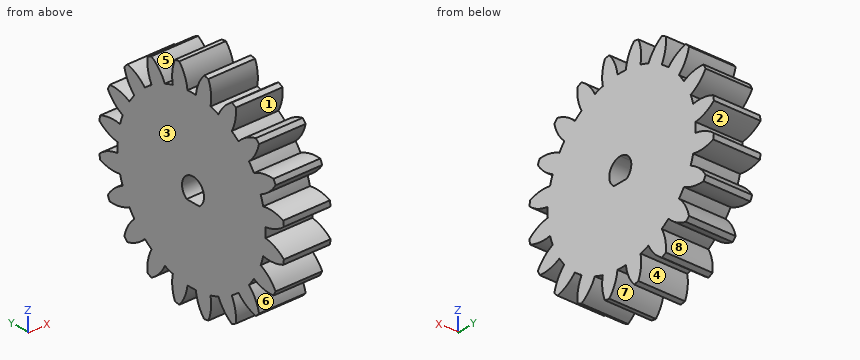
```python
from build123d import *

# Parameters (mm, degrees)
BASPROSKE_W           = 12
BASPROSKE_H           = 27.5
TOOTHCUT_DEPTH        = 41.70012285
TEETHCUTS_COUNT       = 20
TEETHCUTS_ANGLE       = 342
BORSKE_R              = 0.4
BORE_DEPTH            = 50.0000508
KES_EKSTR_ZYON1_DEPTH = 100


with BuildPart() as part:
    # BasProSke → Base-Revolve (revolve)
    with BuildSketch(Plane(origin=(0, 0, 0), x_dir=(1, 0, 0), z_dir=(0, 1, 0)), mode=Mode.PRIVATE) as base_revolve_sk:
        with Locations((6, 13.75)):
            Rectangle(BASPROSKE_W, BASPROSKE_H)
    revolve(base_revolve_sk.sketch.rotate(Axis((-10, 0, 0), (1, 0, 0)), 180), axis=Axis((-10, 0, 0), (1, 0, 0)))

    # TooCutSke → ToothCut (cut, through all)
    with BuildSketch(Plane(origin=(0, 0, 0), x_dir=(0, 0, -1), z_dir=(1, 0, 0))):
        with BuildLine():
            ThreePointArc((1.237725267, 21.838954008), (0, 21.874), (-1.237725267, 21.838954008))
            ThreePointArc((-1.237725267, 21.838954008), (-2.037783758, 24.744650423), (-3.667234079, 27.280011719))
            ThreePointArc((-3.667234079, 27.280011719), (0, 27.5254), (3.667234079, 27.280011719))
            ThreePointArc((3.667234079, 27.280011719), (2.037783758, 24.744650423), (1.237725267, 21.838954008))
        make_face()
    toothcut = extrude(amount=TOOTHCUT_DEPTH, mode=Mode.SUBTRACT)

    # TeethCuts: ToothCut ×20 about axis
    teethcuts_axis = Axis((-10, 0, 0), (1, 0, 0))
    for i in range(1, TEETHCUTS_COUNT):
        add(toothcut.rotate(teethcuts_axis, i * TEETHCUTS_ANGLE / (TEETHCUTS_COUNT - 1)), mode=Mode.SUBTRACT)

    # BorSke → Bore (cut, symmetric)
    with BuildSketch(Plane(origin=(0, 0, 0), x_dir=(0, 0, -1), z_dir=(1, 0, 0))):
        with Locations(Location((0, 0, 0), (0, 0, 180))):
            Circle(BORSKE_R)
    extrude(amount=BORE_DEPTH, both=True, mode=Mode.SUBTRACT)

    # Çizim1 → Kes-Ekstrüzyon1 (cut)
    with BuildSketch(Plane.ZY):
        with BuildLine():
            ThreePointArc((3.25, -0.4), (0.99239773, 2.694777334), (-2.643936459, 1.49))
            Line((-2.643936459, 1.49), (-2.643936459, -2.29))
            ThreePointArc((-2.643936459, -2.29), (0.99239773, -3.494777334), (3.25, -0.4))
        make_face()
    extrude(amount=-KES_EKSTR_ZYON1_DEPTH, mode=Mode.SUBTRACT)


solid = part.part
```
Can you work these out from the model? Positions are in its coordinate system, mm. Face numbers are marked on the shaded views. A direction names the side the tool comes from. Round coordinates to 2 decimals unless told otherwise and drop trailing zeros. Loops run counter-clockwise (first coordinate to the right, second up) from the corner with the lowest first, then second, coordinate; pieces in that order, holes last.
Item 1: Which directions (+Z, -Z, +X, -X, +Y, -Y) give clear straight access to the entire face, cutting with the end or side of a thin tool? Please do the marked faces 5, 6, 7 and 8.
Item 2: Suppose I cut it at B-B, the plane y = 15. Write out the boundary of the cut face in (x, z), then the cut area to 3 significant figures.
Item 3: Please list where these lines run through material, in increasing order: L1, parallel to Y at x = 10.25, z = -17.5; L2, parallel to Z at x = 5.75, y = -23.5; L3, parallel to Z at x = 5, y = 19.
Item 4: Will these pins go through, and if not, where does the flat tip stop? pin 1 Ø3 at (x, z) = (2, -10) entering from -Y; pin 2 Ø5 at (x, z) = (7.5, 14) entering from -Y; pin 3 Ø2 at (y, z) = (21, -2) entering from -X; pin 4 Ø4 at (x, y) = (4, 19.5) entering from +Z.
Item 5: Suppose I cut it at C-C, the plane z = -9. Write out the boundary of the cut face in (x, y), then the cut area to 3 significant figures.
Item 6: If we mould it in two halves opening along Y, with no side actions, what happens to the marked faces 1, 2, 3 and 4? For each: +Y half, -Y half, draft (parallel to the pull), parting line (faces both ways), or undercut.
Item 7: Suppose I cut it at A-A, the plane z = -0.5. Write out the boundary of the cut face in (x, y), then the cut area to 3 significant figures.
Reported:
1. face 5: +Z, +X, -X
1. face 6: +X, -X, -Y
1. face 7: -Z, +X, -X
1. face 8: +X, -X
2. outline: (0, -18.01) - (12, -18.01) - (12, 18.01) - (0, 18.01) - close
2. area: 432 mm2
3. L1: y = -19.45 to -14.4, -13.12 to 13.12, 14.4 to 19.45
3. L2: z = -13.11 to -10.17, -5.76 to -1.58, 1.58 to 5.76, 10.17 to 13.11
3. L3: z = -19.88 to -16.52, -12.15 to 12.15, 16.52 to 19.88
4. pin 1: stops at y = -24.55
4. pin 2: stops at y = -24.8
4. pin 3: stops at x = 0
4. pin 4: stops at z = 19.91
5. outline: (0, -22.19) - (12, -22.19) - (12, 22.19) - (0, 22.19) - close
5. area: 533 mm2
6. face 1: undercut
6. face 2: +Y half
6. face 3: draft
6. face 4: undercut
7. outline: (0, -21.87) - (12, -21.87) - (12, -3.61) - (0, -3.61) - close; (0, 2.81) - (12, 2.81) - (12, 21.87) - (0, 21.87) - close
7. area: 448 mm2
